```python
from build123d import *

# Parameters (mm, degrees)
F0_W     = 55.8020919561
F0_H     = 39.1723364592
F0_R     = 14.0094122965
F1_DEPTH = 12.7
F2_DEPTH = 6.35
F3_R     = 5.08
F4_R     = 5.08
F5_R     = 8.4755986108
F6_DEPTH = 125.9534060955


with BuildPart() as f1:
    # F0 (on Top) → F1 (new body, symmetric)
    with BuildSketch(Plane.XY):
        with BuildLine():
            Line((0, 22.542566061), (-45.4546958208, 22.542566061))
            Line((-45.4546958208, 22.542566061), (-45.4546958208, -27.7162790298))
            Line((-45.4546958208, -27.7162790298), (0, -27.7162790298))
            ThreePointArc((0, -27.7162790298), (37.5493840713, -13.2993479579), (55.8020919561, 22.542566061))
            Line((55.8020919561, 22.542566061), (0, 22.542566061))
        make_face()
        with Locations((27.9010459781, 42.1287342906)):
            Rectangle(F0_W, F0_H)
        with Locations((27.5138542056, 42.0944318175)):
            Circle(F0_R, mode=Mode.SUBTRACT)
    extrude(amount=F1_DEPTH, both=True)

    # F0 (on Top) → F2 (cut, symmetric)
    with BuildSketch(Plane.XY):
        with Locations((27.9010459781, 42.1287342906)):
            Rectangle(F0_W, F0_H)
        with Locations((27.5138542056, 42.0944318175)):
            Circle(F0_R, mode=Mode.SUBTRACT)
    extrude(amount=F2_DEPTH, both=True, mode=Mode.SUBTRACT)

    # F3
    f3_edges = [f1.edges().sort_by_distance(p)[0] for p in [
        (0, 22.542566, 9.525),
    ]]
    fillet(f3_edges, radius=F3_R)

    # F4
    f4_edges = [f1.edges().sort_by_distance(p)[0] for p in [
        (0, 22.542566, -9.525),
    ]]
    fillet(f4_edges, radius=F4_R)

    # F5 (on face) → F6 (cut)
    with BuildSketch(Plane(origin=(-45.4546958208, 0, 0), x_dir=(0, -1, 0), z_dir=(-1, 0, 0))):
        Circle(F5_R)
    extrude(amount=-F6_DEPTH, mode=Mode.SUBTRACT)


solid = f1.part
```
Here's how the part is built. I have some questions about the finished solid (model axes, mm). A direction names the side the tool comes from. Give positions to 0.01 mm unless a question says otherwise; leave off trailing zeros. Order: outer loops, then holes, each group sorted by start corner. A loop starts at its lowest first (then second) coordinate and runs counter-clockwise, first axis right, second up. Notation, with made-up numbers: (-37.5, -33) - (18.5, -33) arc R13 cw to (18.5, -25) - close; hole circle Ø11 at (-27, 48.25). An arc over 180 degrees is marked (long way). Answer as a JSON object with one key per item and string values. Group by question number.
Item 1: If we section it at D-D on y = 0: Please give me the cut outline in (x, z), and give its area (3 significant figures).
Item 2: If we section it at C-C on x = -11.5: Please give me the cut outline in (y, z).
Item 3: If we mould it in two halves opening along X, with no side actions, what happens to faces 1 (the flat face through (0, 44, -9)), 2 (the flat face through (55.802, 42, 10)), 3 (the cylindrical face through (16.396, 33.57, 9.481))? For each: pulls with the +X half, pulls with the -X half, needs draft (parallel to the pull), parting line crosses it, or undercut.
Item 4: Please list where these lines run through material, in increasing order: probe 1 along Z at (x, y) = (-21, 0); probe 2 along Y at (x, z) = (-15.5, 0); probe 3 along Z at (x, y) = (6.5, 55.5).
Item 5: For P1, Ø4, axis at x = 28.5, z = -1, coming from the -Y side; P2, Ø5, axis at x = 4, z = -9.5, coming from the -Y side; P3, Ø22.5, axis at x = 27.51, y = 42.09, coming from the +Z side; P4, Ø3, axis at y = 45, z = -9, coming from the -X side, each with a flat end and sliding along its axis, tell me the tip position at first contact or that it passes through.
Item 6: Which directions (+Z, -Z, +X, -X, +Y, -Y) give clear straight access to the entire face, cutting with the end or side of a thin tool? Please do faces 4 (the flat face through (38.5, 51.1, -6.35)), 5 (the flat face through (0, 44, 10)), 6 (the flat face through (4, 8, 12.7)), 7 (the flat face through (4, 8, -12.7)), 8 (the flat face through (-5, 22.543, 0)).
Item 7: If we section it at B-B on y = 48: Please give me the cut outline in (x, z), and give its area (3 significant figures).
Item 8: If we section it at A-A on z = 0: Please give me the cut outline in (x, y).
Result set:
{
 "1": {"outline": "(-45.45, -12.7) - (48.39, -12.7) - (48.39, -8.48) - (-45.45, -8.48) - close; (-45.45, 8.48) - (48.39, 8.48) - (48.39, 12.7) - (-45.45, 12.7) - close", "area": "793 mm²"},
 "2": {"outline": "(-27.72, -12.7) - (22.54, -12.7) - (22.54, 12.7) - (-27.72, 12.7) - close; hole circle Ø16.95 at (0, 0)"},
 "3": {"face 1": "pulls with the -X half", "face 2": "pulls with the +X half", "face 3": "undercut"},
 "4": {"probe 1": "-12.7 to -8.48, 8.48 to 12.7", "probe 2": "-27.72 to -8.48, 8.48 to 22.54", "probe 3": "-12.7 to -6.35, 6.35 to 12.7"},
 "5": {"P1": "y = -21.06", "P2": "y = -27.7", "P3": "through", "P4": "x = 0"},
 "6": {"face 4": "+X, -X, +Y", "face 5": "+Z, -Z, -X, +Y", "face 6": "+Z, +X, -X, +Y, -Y", "face 7": "-Z, +X, -X, +Y, -Y", "face 8": "-X, +Y"},
 "7": {"outline": "(0, -12.7) - (14.81, -12.7) - (14.81, -6.35) - (0, -6.35) - close; (0, 6.35) - (14.81, 6.35) - (14.81, 12.7) - (0, 12.7) - close; (40.22, -12.7) - (55.8, -12.7) - (55.8, -6.35) - (40.22, -6.35) - close; (40.22, 6.35) - (55.8, 6.35) - (55.8, 12.7) - (40.22, 12.7) - close", "area": "386 mm²"},
 "8": {"outline": "(-45.45, -27.72) - (0, -27.72) arc R56.11 ccw to (42.3, -8.48) - (-45.45, -8.48) - close; (-45.45, 8.48) - (52.45, 8.48) arc R56.11 ccw to (55.8, 22.54) - (-45.45, 22.54) - close"}
}
